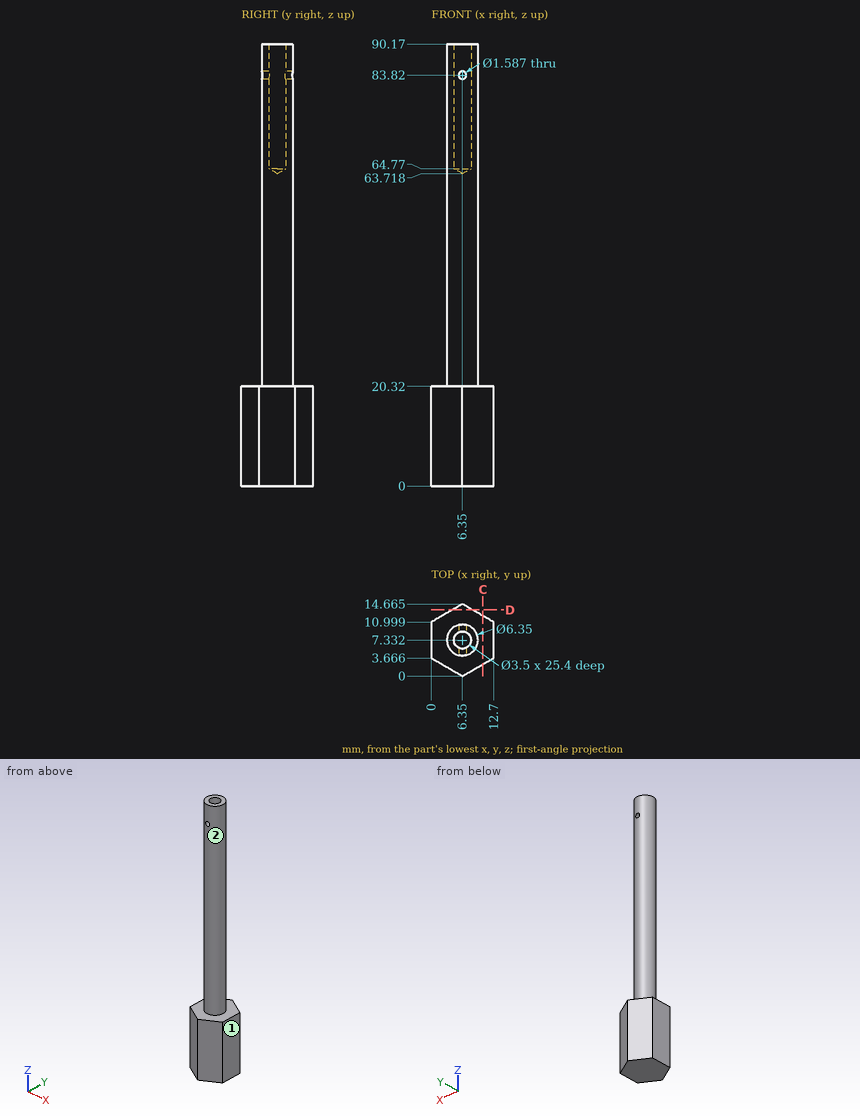
Here's the drawing with two shaded views (mm, measured from the low corner). I have some questions. A direction names the side the tool comes from. Coordinates: 2 decimals unless noted, no trailing zeros. Write each loop counter-clockwise with the first axis right and the second up, starting at its lowest first coordinate (ties: lowest second). Pieces come first, ordered by that corner, then holes.
Item 1: I want a section at C-C on x = 10.5. Write out the boundary of the cut face in (y, z) (1 decimal).
Item 2: On a 3-axis mill with a long thin cutter (end or side, diameter ignored), from which of +Z, -Z, +X, -X, +Y, -Y can I reach the whole of each face in a straight line? I mean the marked faces 1 and 2. Say none if no direction works.
Item 3: I want a section at D-D on y = 13.5. Write out the boundary of the cut face in (x, z).
Item 4: If I drill on line 1 (Z direction, x = 6.5, y = 4.5); line 2 (Y direction, x = 6.35, z = 77); line 3 (Y direction, x = 4.75, z = 68) (1 decimal), over which ranges is the centre line in solid material (lowest first)?
Item 5: Will these pins go through, and if not, where does the flat tip stop? pin 1 (1 mm diameter, centred on x = 6.35, z = 83.82, fed in from -Y); pin 2 (4 mm diameter, centred on x = 5, z = 51.5, fed in from +Y); pin 3 (2 mm diameter, centred on x = 6.35, z = 83.82, fed in from -Y); pin 4 (5 mm diameter, centred on x = 2, z = 77.5, fed in from -Y).
Findings below:
1. outline: (2.4, 0) - (12.3, 0) - (12.3, 20.3) - (2.4, 20.3) - close
2. face 1: +Z, -Z, +X, +Y, -Y
2. face 2: +Z
3. outline: (4.33, 0) - (8.37, 0) - (8.37, 20.32) - (4.33, 20.32) - close
4. line 1: z = 0 to 83.04, 84.6 to 90.17
4. line 2: y = 4.16 to 5.58, 9.08 to 10.51
4. line 3: y = 4.6 to 6.6, 8 to 10.1
5. pin 1: passes through
5. pin 2: stops at y = 10.51
5. pin 3: stops at y = 4.16
5. pin 4: stops at y = 4.75
